Check sheet for the modelled part. Datum: model origin and axes. Units: mm. A direction names the side the tool comes from. Give positions to 0.01 mm unless a question says otherwise; leave off trailing zeros. Write each loop counter-clockwise with the first axis right and the second up, starting at its lowest first coordinate (ties: lowest second). Pieces come first, ordered by that corner, then holes. Notation, with made-up numbers: M -5.75,12 L 21.25,12 A27 ccw 21.25,32 Z; hole C 73.25,-24 d3. An arc over 180 degrees is marked long. Write item = value, one per line. Start each with the question number.
1) Scan lines: L1, parallel to X at y = 2, z = -29.5; L2, parallel to X at y = 9.85, z = 29.5; L3, parallel to Z at x = -24.5, y = 15. Record each from-to range of solid material in increasing order.
2) Set-up check for faces 1 (the face through (32.1, 7.5, 31)), 2 (the face through (1, 0, -1)), 3 (the face through (-29.6, 9.4, -24.5)): record each of +Z, -Z, +X, -X, +Y, -Y from which the full face is reachable in a straight line by a thin tool's end or side.
3) Draft check along X on faces 4 (the face through (29.45, 9, 27.56)), 5 (the face through (-37.5, 12, 0)), 6 (the face through (37.5, 12, 0)). Enter one of: pulls with the +X half, pulls with the -X half, needs draft (parallel to the pull), parting line crosses it, or undercut.
4) Sectioned sample at D-D, the plane x = -29.5. Count the separate pieces of the cut face and the enclosed holes in it, then the cut area to 3 significant figures.
5) Sectioned sample at C-C, the plane z = 8. Record the cut outline in (x, y).
6) Sectioned sample at B-B, the plane x = 16.25. Record the cut outline in (y, z), then the cut area to 3 significant figures.
7) Sectioned sample at A-A, the plane x = -12.5. Record the cut outline in (y, z), then the cut area to 3 significant figures.
8) Gauge pin test, flat ends, axial feed: pin 1 (2 mm diameter, centred on x = -23, z = -0.5, fed in from +Y); pin 2 (4 mm diameter, centred on x = 7, z = -28, fed in from +Y); pin 3 (2 mm diameter, centred on x = 31, z = 26.5, fed in from +Y). Record the tip position at first contact, or that the pin passes through.
from build123d import *

# Parameters (mm, degrees)
SKETCH_1_W          = 75
SKETCH_1_H          = 75
EXTRUDE_1_DEPTH     = 25
SHELL_1_T           = -3
SKETCH_3_W          = 10
SKETCH_3_H          = 10
EXTRUDE_2_DEPTH     = 9
CUT_EXTRUDE_1_REACH = 56.603
SKETCH_4_R          = 1.75
CUT_EXTRUDE_START   = -3
CUT_EXTRUDE_2_DEPTH = 3
CUT_EXTRUDE_3_REACH = 89.5
SKETCH_6_R          = 6
SKETCH_6_R_2        = 2.5
EXTRUDE_3_DEPTH     = 10
SKETCH_8_R          = 1
CUT_EXTRUDE_4_DEPTH = 4
FILLET_1_R          = 4
FILLET_2_R          = 1


with BuildPart() as part:
    # 草图1 → 凸台-拉伸1 (new body)
    with BuildSketch(Plane(origin=(0, 0, 0), x_dir=(1, 0, 0), z_dir=(0, 1, 0))):
        Rectangle(SKETCH_1_W, SKETCH_1_H)
    extrude(amount=EXTRUDE_1_DEPTH)

    # 抽壳1
    shell_1_openings = [part.faces().sort_by_distance(p)[0] for p in [
        (0, 25, 0),
    ]]
    offset(amount=SHELL_1_T, openings=shell_1_openings, kind=Kind.INTERSECTION)

    # 草图3 → 凸台-拉伸2 (add)
    with BuildSketch(Plane(origin=(0, 3, 0), x_dir=(1, 0, 0), z_dir=(0, 1, 0))):
        with Locations((-29.5, -29.5)):
            Rectangle(SKETCH_3_W, SKETCH_3_H)
        with Locations((29.5, -29.5)):
            Rectangle(SKETCH_3_W, SKETCH_3_H)
        with Locations((29.5, 29.5)):
            Rectangle(SKETCH_3_W, SKETCH_3_H)
        with Locations((-29.5, 29.5)):
            Rectangle(SKETCH_3_W, SKETCH_3_H)
    extrude(amount=EXTRUDE_2_DEPTH)

    # 草图4 → 切除-拉伸1 (cut, up to next)
    with BuildSketch(Plane(origin=(0, 12, 0), x_dir=(1, 0, 0), z_dir=(0, 1, 0)), mode=Mode.PRIVATE) as cut_extrude_1_sk1:
        with Locations(Location((-29.5, 29.5, 0), (0, 0, 270))):
            Circle(SKETCH_4_R)
    cut_extrude_1_tool1 = extrude(cut_extrude_1_sk1.sketch, amount=-CUT_EXTRUDE_1_REACH, mode=Mode.PRIVATE) & part.part
    # 草图4 → 切除-拉伸1 (cut, up to next)
    with BuildSketch(Plane(origin=(0, 12, 0), x_dir=(1, 0, 0), z_dir=(0, 1, 0)), mode=Mode.PRIVATE) as cut_extrude_1_sk2:
        with Locations(Location((29.5, 29.5, 0), (0, 0, 270))):
            Circle(SKETCH_4_R)
    cut_extrude_1_tool2 = extrude(cut_extrude_1_sk2.sketch, amount=-CUT_EXTRUDE_1_REACH, mode=Mode.PRIVATE) & part.part
    # 草图4 → 切除-拉伸1 (cut, up to next)
    with BuildSketch(Plane(origin=(0, 12, 0), x_dir=(1, 0, 0), z_dir=(0, 1, 0)), mode=Mode.PRIVATE) as cut_extrude_1_sk3:
        with Locations(Location((29.5, -29.5, 0), (0, 0, 270))):
            Circle(SKETCH_4_R)
    cut_extrude_1_tool3 = extrude(cut_extrude_1_sk3.sketch, amount=-CUT_EXTRUDE_1_REACH, mode=Mode.PRIVATE) & part.part
    # 草图4 → 切除-拉伸1 (cut, up to next)
    with BuildSketch(Plane(origin=(0, 12, 0), x_dir=(1, 0, 0), z_dir=(0, 1, 0)), mode=Mode.PRIVATE) as cut_extrude_1_sk4:
        with Locations(Location((-29.5, -29.5, 0), (0, 0, 270))):
            Circle(SKETCH_4_R)
    cut_extrude_1_tool4 = extrude(cut_extrude_1_sk4.sketch, amount=-CUT_EXTRUDE_1_REACH, mode=Mode.PRIVATE) & part.part
    add(cut_extrude_1_tool1.solids().sort_by_distance((-29.5, 12, -29.5))[0], mode=Mode.SUBTRACT)
    add(cut_extrude_1_tool2.solids().sort_by_distance((29.5, 12, -29.5))[0], mode=Mode.SUBTRACT)
    add(cut_extrude_1_tool3.solids().sort_by_distance((29.5, 12, 29.5))[0], mode=Mode.SUBTRACT)
    add(cut_extrude_1_tool4.solids().sort_by_distance((-29.5, 12, 29.5))[0], mode=Mode.SUBTRACT)

    # 草图5 → 切除-拉伸2 (cut)
    with BuildSketch(Plane(origin=(0, 12, 0), x_dir=(1, 0, 0), z_dir=(0, 1, 0)).offset(CUT_EXTRUDE_START)):
        Polygon((-26.035898385, 29.5), (-27.767949192, 32.5), (-31.232050808, 32.5), (-32.964101615, 29.5), (-32.964101615, 24.5), (-26.035898385, 24.5), align=None)
        Polygon((32.964101615, 29.5), (31.232050808, 32.5), (27.767949192, 32.5), (26.035898385, 29.5), (26.035898385, 24.5), (32.964101615, 24.5), align=None)
        Polygon((26.035898385, -29.5), (27.767949192, -32.5), (31.232050808, -32.5), (32.964101615, -29.5), (32.964101615, -24.5), (26.035898385, -24.5), align=None)
        Polygon((-32.964101615, -29.5), (-31.232050808, -32.5), (-27.767949192, -32.5), (-26.035898385, -29.5), (-26.035898385, -24.5), (-32.964101615, -24.5), align=None)
    extrude(amount=-CUT_EXTRUDE_2_DEPTH, mode=Mode.SUBTRACT)

    # 草图6 → 切除-拉伸3 (cut, up to next)
    with BuildSketch(Plane(origin=(0, 0, -37.5), x_dir=(-1, 0, 0), z_dir=(0, 0, -1)), mode=Mode.PRIVATE) as cut_extrude_3_sk1:
        with Locations((12.5, 14)):
            Circle(SKETCH_6_R)
    cut_extrude_3_tool1 = extrude(cut_extrude_3_sk1.sketch, amount=-CUT_EXTRUDE_3_REACH, mode=Mode.PRIVATE) & part.part
    # 草图6 → 切除-拉伸3 (cut, up to next)
    with BuildSketch(Plane(origin=(0, 0, -37.5), x_dir=(-1, 0, 0), z_dir=(0, 0, -1)), mode=Mode.PRIVATE) as cut_extrude_3_sk2:
        with Locations((-12.5, 14)):
            Circle(SKETCH_6_R_2)
    cut_extrude_3_tool2 = extrude(cut_extrude_3_sk2.sketch, amount=-CUT_EXTRUDE_3_REACH, mode=Mode.PRIVATE) & part.part
    add(cut_extrude_3_tool1.solids().sort_by_distance((-12.5, 14, -37.5))[0], mode=Mode.SUBTRACT)
    add(cut_extrude_3_tool2.solids().sort_by_distance((12.5, 14, -37.5))[0], mode=Mode.SUBTRACT)

    # 草图7 → 凸台-拉伸3 (add)
    with BuildSketch(Plane.XY.offset(-34.5)):
        with BuildLine():
            Line((20, 0), (5, 0))
            Line((5, 0), (5, 14))
            Line((5, 14), (11.5, 14))
            ThreePointArc((11.5, 14), (12.5, 13), (13.5, 14))
            Line((13.5, 14), (20, 14))
            Line((20, 14), (20, 0))
        make_face()
    extrude(amount=EXTRUDE_3_DEPTH)

    # 草图8 → 切除-拉伸4 (cut)
    with BuildSketch(Plane(origin=(0, 14, 0), x_dir=(1, 0, 0), z_dir=(0, 1, 0))):
        with Locations(Location((16.25, 29.5, 0), (0, 0, 180))):
            Circle(SKETCH_8_R)
        with Locations(Location((8.75, 29.5, 0), (0, 0, 180))):
            Circle(SKETCH_8_R)
    extrude(amount=-CUT_EXTRUDE_4_DEPTH, mode=Mode.SUBTRACT)

    # 圆角1
    fillet_1_edges = [part.edges().sort_by_distance(p)[0] for p in [
        (34.5, 18.5, 34.5),
        (34.5, 18.5, -34.5),
        (-34.5, 18.5, -34.5),
        (-34.5, 18.5, 34.5),
        (37.5, 12.5, 37.5),
        (-37.5, 12.5, 37.5),
        (-37.5, 12.5, -37.5),
        (37.5, 12.5, -37.5),
    ]]
    fillet(fillet_1_edges, radius=FILLET_1_R)

    # 圆角2
    fillet_2_edges = [part.edges().sort_by_distance(p)[0] for p in [
        (20, 8.5, -34.5),
        (5, 8.5, -34.5),
        (5, 8.5, -24.5),
        (20, 8.5, -24.5),
        (-34.5, 12, -27.5),
        (-27.5, 12, 34.5),
        (-33.328427125, 12, 33.328427125),
        (27.5, 12, -34.5),
        (-33.328427125, 12, -33.328427125),
        (34.5, 12, 27.5),
        (33.328427125, 12, 33.328427125),
        (33.328427125, 12, -33.328427125),
        (-34.5, 7.5, -24.5),
        (-24.5, 7.5, -24.5),
        (-24.5, 7.5, -34.5),
        (-27.5, 12, -34.5),
        (-34.5, 7.5, 24.5),
        (-24.5, 7.5, 34.5),
        (-24.5, 7.5, 24.5),
        (-34.5, 12, 27.5),
        (34.5, 7.5, 24.5),
        (24.5, 7.5, 24.5),
        (24.5, 7.5, 34.5),
        (27.5, 12, 34.5),
        (34.5, 7.5, -24.5),
        (24.5, 7.5, -34.5),
        (24.5, 7.5, -24.5),
        (34.5, 12, -27.5),
    ]]
    fillet(fillet_2_edges, radius=FILLET_2_R)


solid = part.part
Data:
q1.L1 = -37.5 to -31.25, -27.75 to 27.75, 31.25 to 37.5
q1.L2 = -37.5 to -31.25, -27.75 to -24.5, 24.5 to 27.75, 31.25 to 37.5
q1.L3 = -37.5 to -34.5, 34.5 to 37.5
q2.face_1 = none
q2.face_2 = +Z, -Z, +X, -X, -Y
q2.face_3 = +Y
q3.face_4 = undercut
q3.face_5 = pulls with the -X half
q3.face_6 = pulls with the +X half
q4.separate_pieces = 5
q4.enclosed_holes = 0
q4.area = 426 mm2
q5.outline = M -37.5,0 L 37.5,0 L 37.5,25 L 34.5,25 L 34.5,3 L -34.5,3 L -34.5,25 L -37.5,25 Z
q6.outline = M 0,-37.5 L 25,-37.5 L 25,-34.5 L 14,-34.5 L 14,-30.5 L 10,-30.5 L 10,-28.5 L 14,-28.5 L 14,-24.5 L 3,-24.5 L 3,34.5 L 25,34.5 L 25,37.5 L 0,37.5 Z
q6.area = 459 mm2
q7.outline = M 0,-37.5 L 8,-37.5 L 8,-34.5 L 3,-34.5 L 3,34.5 L 25,34.5 L 25,37.5 L 0,37.5 Z; M 20,-37.5 L 25,-37.5 L 25,-34.5 L 20,-34.5 Z
q7.area = 321 mm2
q8.pin_1 = 3
q8.pin_2 = 14
q8.pin_3 = 12
